```python
from build123d import *

# Parameters (mm, degrees)
F0_W     = 292.1
F0_H     = 241.3
F0_W_2   = 76.2
F0_H_2   = 63.5
F1_DEPTH = 21.59
F2_DEPTH = 2.54
F3_W     = 38.1
F3_H     = 11.9225998908
F3_W_2   = 12.7
F3_H_2   = 38.1
F3_H_3   = 12.7
F3_H_4   = 13.060019505
F3_H_5   = 12.339980495
F3_W_3   = 13.0705659449
F4_DEPTH = 5.08


with BuildPart() as f1:
    # F0 (on Top) → F1 (new body)
    with BuildSketch(Plane.XY):
        with Locations((-4.8260282278, 1.4313216329)):
            Rectangle(F0_W, F0_H)
        with Locations((-93.7260282278, -74.4086588621)):
            Rectangle(F0_W_2, F0_H_2, mode=Mode.SUBTRACT)
        with Locations((-5.1965941727, -74.7686783671)):
            Rectangle(F0_W_2, F0_H_2, mode=Mode.SUBTRACT)
        with Locations((84.0739717722, -74.4086588621)):
            Rectangle(F0_W_2, F0_H_2, mode=Mode.SUBTRACT)
        Polygon((-42.9260282278, -30.3186783671), (-42.9260282278, 9.6084550023), (-42.9260282278, 33.1813216329), (33.2739717722, 33.1813216329), (33.2739717722, -30.3186783671), align=None, mode=Mode.SUBTRACT)
        with Locations((84.0739717722, 1.4313216329)):
            Rectangle(F0_W_2, F0_H_2, mode=Mode.SUBTRACT)
        Polygon((-131.8260282278, 33.958721742), (-55.6260282278, 33.958721742), (-55.6260282278, 9.6084550023), (-55.6260282278, -29.541278258), (-131.8260282278, -29.541278258), align=None, mode=Mode.SUBTRACT)
        with Locations((-93.7260282278, 77.6313216329)):
            Rectangle(F0_W_2, F0_H_2, mode=Mode.SUBTRACT)
        with Locations((-4.8260282278, 77.6313216329)):
            Rectangle(F0_W_2, F0_H_2, mode=Mode.SUBTRACT)
        with Locations((84.0739714861, 77.6313216329)):
            Rectangle(F0_W_2, F0_H_2, mode=Mode.SUBTRACT)
    extrude(amount=F1_DEPTH)

    # F0 (on Top) → F2 (join)
    with BuildSketch(Plane.XY):
        with Locations((-4.8260282278, 77.6313216329)):
            Rectangle(F0_W_2, F0_H_2)
        Polygon((-42.9260282278, 33.1813216329), (-42.9260282278, 9.6084550023), (-42.9260282278, -30.3186783671), (33.2739717722, -30.3186783671), (33.2739717722, 33.1813216329), align=None)
        with Locations((-5.1965941727, -74.7686783671)):
            Rectangle(F0_W_2, F0_H_2)
        Polygon((-55.6260282278, 9.6084550023), (-55.6260282278, 33.958721742), (-131.8260282278, 33.958721742), (-131.8260282278, -29.541278258), (-55.6260282278, -29.541278258), align=None)
        with Locations((84.0739717722, 1.4313216329)):
            Rectangle(F0_W_2, F0_H_2)
    extrude(amount=F2_DEPTH)

    # F3 (on face) → F4 (cut)
    with BuildSketch(Plane.XY.offset(21.59)):
        with Locations((-74.6390915036, 39.9200216874)):
            Rectangle(F3_W, F3_H)
        with Locations((-49.2760282278, 70.8251611769)):
            Rectangle(F3_W_2, F3_H_2)
        with Locations((-15.7696923733, 39.5313216329)):
            Rectangle(F3_W, F3_H_3)
        with Locations((-82.3410557747, 115.7313216329)):
            Rectangle(F3_W_2, F3_H_3)
        with Locations((92.96223948, -112.6886686146)):
            Rectangle(F3_W_2, F3_H_4)
        with Locations((73.1869616985, -36.4886686146)):
            Rectangle(F3_W, F3_H_5)
        with Locations((39.4386887997, -77.696109426)):
            Rectangle(F3_W_3, F3_H_2)
    extrude(amount=-F4_DEPTH, mode=Mode.SUBTRACT)


solid = f1.part
```
Can you work these out from the model? Positions are in its coordinate system, mm. A direction names the side the tool comes from. Give positions to 0.01 mm unless a question says otherwise; leave off trailing zeros. Loops run counter-clockwise (first coordinate to the right, second up) from the corner with the lowest first, then second, coordinate; pieces in that order, holes last. Notation, with made-up numbers: M 78,-36.5 L 110,-36.5 A19 ccw 110,-17.5 Z; hole C 15.5,-30 d9. An arc over 180 degrees is marked long. Use CSV: the item, a comma, the result in double quotes. Start each with the question number.
1. If I drill on L1, parallel to Y at x = 102, z = 17; L2, parallel to X at y = -51, z = 6; L3, parallel to Y at x = -29, z = 3.25, over which ranges is the centre line in solid material (lowest first)?
2. Imagine slicing it at B-B, the plane y = 25. Write out the boundary of the cut face in (x, z).
3. Imagine slicing it at A-A, the plane x = -101. Write out the boundary of the cut face in (y, z), plus the area to 3 significant figures.
4. Imagine slicing it at D-D, the plane x = -65. Write out the boundary of the cut face in (y, z).
5. If we mould it in two halves opening along X, with no side actions, what happens to faces 1 (the face through (-7, 122.081, 11)), 2 (the face through (-42.926, 1, 12)), 3 (the face through (-150.876, 0, 11))? For each: released by +X, released by -X, zero draft, split by the parting line, or undercut.
6. For P1, Ø3.5, axis at x = -74, y = 38, coming from the +Z side, with a flat end and sliding along its axis, tell me the tip position at first contact or that it passes through.
7. Imagine slicing it at C-C, the plane z = 11.75. Count the separate pieces of the cut face and the enclosed holes in it, plus the area to 3 significant figures.
8. On a 3-axis mill with a long thin cutter (end or side, diameter ignored), from which of +Z, -Z, +X, -X, +Y, -Y can I reach the whole of each face in a straight line? I mean faces 4 (the face through (84, -42.659, 11)), 5 (the face through (-5, 78, 2.54)), 6 (the face through (-16, -34, 21.59)), 7 (the face through (93, -113, 16.51)). Say none if no direction works.
Response values:
1,L1,"-119.22 to -106.16, -42.66 to -30.32, 33.18 to 45.88, 109.38 to 122.08"
1,L2,"-150.88 to -131.83, -55.63 to -43.3, 32.9 to 45.97, 122.17 to 141.22"
1,L3,"-119.22 to -106.52, -43.02 to -30.32, 33.18 to 45.88, 109.38 to 122.08"
2,outline,"M -150.88,0 L 141.22,0 L 141.22,21.59 L 122.17,21.59 L 122.17,2.54 L 45.97,2.54 L 45.97,21.59 L 33.27,21.59 L 33.27,2.54 L -42.93,2.54 L -42.93,21.59 L -55.63,21.59 L -55.63,2.54 L -131.83,2.54 L -131.83,21.59 L -150.88,21.59 Z"
3,outline,"M -119.22,0 L -106.16,0 L -106.16,21.59 L -119.22,21.59 Z; M -42.66,0 L 45.88,0 L 45.88,21.59 L 33.96,21.59 L 33.96,2.54 L -29.54,2.54 L -29.54,21.59 L -42.66,21.59 Z; M 109.38,0 L 122.08,0 L 122.08,21.59 L 109.38,21.59 Z"
3,area,"1,260 mm^2"
4,outline,"M -119.22,0 L -106.16,0 L -106.16,21.59 L -119.22,21.59 Z; M -42.66,0 L 45.88,0 L 45.88,16.51 L 33.96,16.51 L 33.96,2.54 L -29.54,2.54 L -29.54,21.59 L -42.66,21.59 Z; M 109.38,0 L 122.08,0 L 122.08,21.59 L 109.38,21.59 Z"
5,face 1,"zero draft"
5,face 2,"undercut"
5,face 3,"released by -X"
6,P1,"z = 16.51"
7,separate pieces,"1"
7,enclosed holes,"9"
7,area,"26,900 mm^2"
8,face 4,"+Z, -Z"
8,face 5,"+Z"
8,face 6,"+Z, +X, -X, +Y, -Y"
8,face 7,"+Z, -Y"
